Here's how the part is built. I have some questions about the finished solid (model axes, mm). Face numbers are marked on the shaded views. A direction names the side the tool comes from. Give positions to 0.01 mm unless a question says otherwise; leave off trailing zeros. Write each loop counter-clockwise with the first axis right and the second up, starting at its lowest first coordinate (ties: lowest second). Pieces come first, ordered by that corner, then holes. Notation, with made-up numbers: (-27.5, 80.5) - (9.5, 80.5) arc R22 cw to (9.5, 104.5) - close; hole circle Ø1 at (-2.75, 2.25). An arc over 180 degrees is marked (long way). One line per item, written item: value. Start each with the question number.
1) Imagine slicing it at B-B on z = 16.25. Write out the boundary of the cut face in (x, y).
2) Imagine slicing it at D-D on x = 3.75. Write out the boundary of the cut face in (y, z).
3) Please list where these lines run through material, in increasing order: L1, parallel to Y at x = 0, z = 3; L2, parallel to Y at x = 0, z = 15; L3, parallel to Z at x = -4, y = 4.5. Write a range as [from, to].
4) Imagine slicing it at A-A on x = 0. Write out the boundary of the cut face in (y, z).
5) Imagine slicing it at C-C on y = -3.25. Write out the boundary of the cut face in (x, z).
6) I'm going to push flat-ended pins straight in: P1, Ø1, axis at y = -2.5, z = 7.5, coming from the -X side; P2, Ø1.5, axis at x = -5, z = 8.5, coming from the -Y side; P3, Ø2.5, axis at x = 0, y = 0, coming from the -Z side; P4, Ø1.5, axis at x = -4.5, z = 5.5, coming from the +Y side. Where does each tip first touch, or does it pass through?
7) We'd pull the mould along X, two halves only. Please class the marked faces 1, 2, 3 and 4: +X half, -X half, draft (parallel to the pull), parting line (faces both ways), or undercut.
8) On a 3-axis mill with a long thin cutter (end or side, diameter ignored), from which of +Z, -Z, +X, -X, +Y, -Y can I reach the whole of each face in a straight line? I mean the marked faces 5 and 6. Say none if no direction works.
from build123d import *

# Parameters (mm, degrees)
TAP_DRILL_FOR_M4X0_7_TAP1_D     = 3.3
TAP_DRILL_FOR_M4X0_7_TAP1_DEPTH = 5
TAP_DRILL_FOR_M4X0_7_TAP1_TIP   = 0.991420021
SKETCH9_OUTSIDE_W               = 25.62
SKETCH9_OUTSIDE_H               = 25.62
CUT_EXTRUDE1_DEPTH              = 22.843191159


with BuildPart() as part:
    # Sketch1 → Revolve1 (revolve)
    with BuildSketch(Plane(origin=(0, 0, 0), x_dir=(0, 0, -1), z_dir=(1, 0, 0)), mode=Mode.PRIVATE) as revolve1_sk:
        Polygon((0, -2), (0, -5.75), (-13, -5.75), (-13, -8.75), (-18, -8.75), (-18, 0), (-13, 0), (-13, -2), align=None)
    revolve(revolve1_sk.sketch.rotate(Axis((0, 0, 36.965240676), (0, 0, -1)), 270), axis=Axis((0, 0, 36.965240676), (0, 0, -1)))

    # Tap Drill for M4x0.7 Tap1
    with Locations(Plane.XY.offset(18)):
        with Locations((0, 0)):
            Hole(TAP_DRILL_FOR_M4X0_7_TAP1_D / 2, depth=TAP_DRILL_FOR_M4X0_7_TAP1_DEPTH)
            with Locations((0, 0, -(TAP_DRILL_FOR_M4X0_7_TAP1_DEPTH + TAP_DRILL_FOR_M4X0_7_TAP1_TIP / 2))):  # 118° drill point
                Cone(0, TAP_DRILL_FOR_M4X0_7_TAP1_D / 2, TAP_DRILL_FOR_M4X0_7_TAP1_TIP, mode=Mode.SUBTRACT)

    # Sketch9 outside → Cut-Extrude1 (cut, through all)
    with BuildSketch(Plane.XY.offset(18)):
        Rectangle(SKETCH9_OUTSIDE_W, SKETCH9_OUTSIDE_H)
        Polygon((3.464101615, -6), (6.92820323, 0), (3.464101615, 6), (-3.464101615, 6), (-6.92820323, 0), (-3.464101615, -6), align=None, mode=Mode.SUBTRACT)
    extrude(amount=-CUT_EXTRUDE1_DEPTH, mode=Mode.SUBTRACT)


solid = part.part
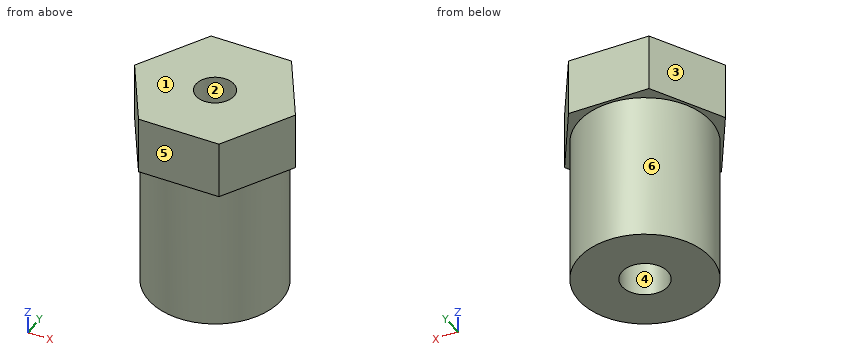
Numbers:
1. outline: (-6.93, 0) - (-3.46, -6) - (3.46, -6) - (6.93, 0) - (3.46, 6) - (-3.46, 6) - close; hole circle Ø3.3 at (0, 0)
2. outline: (-5.5, 13) - (-4.36, 13) - (-4.36, 0) - (4.36, 0) - (4.36, 13) - (5.5, 13) - (5.5, 18) - (-5.5, 18) - close
3. L1: [-5.75, -2], [2, 5.75]
3. L2: [-6, -1.65], [1.65, 6]
3. L3: [13, 18]
4. outline: (-6, 13) - (-5.75, 13) - (-5.75, 0) - (-2, 0) - (-2, 13) - (-1.65, 13) - (-1.65, 18) - (-6, 18) - close; (1.65, 13) - (2, 13) - (2, 0) - (5.75, 0) - (5.75, 13) - (6, 13) - (6, 18) - (1.65, 18) - close
5. outline: (-5.05, 13) - (-4.74, 13) - (-4.74, 0) - (4.74, 0) - (4.74, 13) - (5.05, 13) - (5.05, 18) - (-5.05, 18) - close
6. P1: x = -5.39
6. P2: y = -3.87
6. P3: through
6. P4: y = 4.36
7. face 1: draft
7. face 2: undercut
7. face 3: -X half
7. face 4: undercut
8. face 5: +Z, -Z, +X, -X, -Y
8. face 6: -Z
